The listing builds one solid part. Answer for the finished solid, in the listing's coordinates (mm). A direction names the side the tool comes from. Round coordinates to 2 decimals unless told otherwise and drop trailing zeros. Loops run counter-clockwise (first coordinate to the right, second up) from the corner with the lowest first, then second, coordinate; pieces in that order, holes last. Notation, with made-up numbers: M -17,28.25 L 40,28.25 A13 ccw 40,51.25 Z; hole C 83,34.25 d11. An arc over 180 degrees is marked long. Put each result on its own line as item: value. Start each with the question number.
(1) Section C-C, the plane x = 205.25 is taken. Determine the outline of the cut face in (y, z), then the cut area to 3 significant figures.
(2) Section A-A, the plane z = 1.1 is taken. Count the separate pieces of the cut face and the enclosed holes in it, then the cut area to 3 significant figures.
(3) Determine the mould class of faces 1 (the face through (208.65, 84.93, 1.48)), 2 (the face through (208.556, 171.916, 1.479)), 3 (the face through (204.251, 140, 1)) for opening direction Y: released by +Y, released by -Y, zero draft, split by the parting line, or undercut.
(4) Flat-ended cylindrical pins translate along their axes: P1, Ø4, axis at x = 208.75, y = 98.43, coming from the -Z side; P2, Ø2.5, axis at x = 208.75, y = 152.43, coming from the -Z side. Find the tip coordinate at first contact, or state that the pin passes through.
(5) Which of the six approach directions +Z, -Z, +X, -X, +Y, -Y give full straight-line access (tool end or side, diameter ignored) to faces 4 (the face through (207.251, 139, 1)), 5 (the face through (207, 140, 0))?
(6) Straight lines are drawn through the part: line 1 (X direction, y = 141.5, z = 2.2); line 2 (X direction, y = 125, z = 2.85); line 3 (Y direction, x = 211, z = 1.25). For each, find the intervals that lie inside material, in ascending order.
(7) Section B-B, the plane x = 211.75 is taken. Determine the outline of the cut face in (y, z).
```python
from build123d import *

# Parameters (mm, degrees)
MODEL_R                 = 1.5
SALIENTE_EXTRUIR1_DEPTH = 3


with BuildPart() as part:
    # Model → Saliente-Extruir1 (new body)
    with BuildSketch(Plane.XY):
        with BuildLine():
            Line((213.25077615, 89.428489513), (213.25077615, 188.428489513))
            ThreePointArc((213.25077615, 188.428489513), (208.75077615, 192.928489513), (204.25077615, 188.428489513))
            Line((204.25077615, 188.428489513), (204.25077615, 89.428489513))
            ThreePointArc((204.25077615, 89.428489513), (208.75077615, 84.928489513), (213.25077615, 89.428489513))
        make_face()
        with Locations((208.75077615, 179.428489513)):
            Circle(MODEL_R, mode=Mode.SUBTRACT)
        with Locations((208.75077615, 188.428489513)):
            Circle(MODEL_R, mode=Mode.SUBTRACT)
        with Locations((208.75077615, 152.428489513)):
            Circle(MODEL_R, mode=Mode.SUBTRACT)
        with Locations((208.75077615, 161.428489513)):
            Circle(MODEL_R, mode=Mode.SUBTRACT)
        with Locations((208.75077615, 170.428489513)):
            Circle(MODEL_R, mode=Mode.SUBTRACT)
        with Locations((208.75077615, 116.428489513)):
            Circle(MODEL_R, mode=Mode.SUBTRACT)
        with Locations((208.75077615, 125.428489513)):
            Circle(MODEL_R, mode=Mode.SUBTRACT)
        with Locations((208.75077615, 89.428489513)):
            Circle(MODEL_R, mode=Mode.SUBTRACT)
        with Locations((208.75077615, 98.428489513)):
            Circle(MODEL_R, mode=Mode.SUBTRACT)
        with Locations((208.75077615, 107.428489513)):
            Circle(MODEL_R, mode=Mode.SUBTRACT)
        with BuildLine():
            Line((207.25077615, 134.428489513), (207.25077615, 143.428489513))
            ThreePointArc((207.25077615, 143.428489513), (208.75077615, 144.928489513), (210.25077615, 143.428489513))
            Line((210.25077615, 143.428489513), (210.25077615, 134.428489513))
            ThreePointArc((210.25077615, 134.428489513), (208.75077615, 132.928489513), (207.25077615, 134.428489513))
        make_face(mode=Mode.SUBTRACT)
    extrude(amount=SALIENTE_EXTRUIR1_DEPTH)


solid = part.part
```
Recorded:
1. outline: M 86.6,0 L 191.26,0 L 191.26,3 L 86.6,3 Z
1. area: 314 mm²
2. separate pieces: 1
2. enclosed holes: 11
2. area: 850 mm²
3. face 1: released by -Y
3. face 2: undercut
3. face 3: zero draft
4. P1: stops at z = 0
4. P2: passes through
5. face 4: +Z, -Z
5. face 5: -Z, +X, -X, +Y, -Y
6. line 1: x = 204.25 to 207.25, 210.25 to 213.25
6. line 2: x = 204.25 to 207.31, 210.19 to 213.25
6. line 3: y = 85.53 to 192.33
7. outline: M 86.07,0 L 191.78,0 L 191.78,3 L 86.07,3 Z
